Design review of the part built by this model. Coordinates are the model's own, in mm. Face numbers are marked on the shaded views. Give positions to 0.01 mm unless a question says otherwise; leave off trailing zeros. Order: outer loops, then holes, each group sorted by start corner. A loop starts at its lowest first (then second) coordinate and runs counter-clockwise, first axis right, second up. Notation, with made-up numbers: (61, 24.25) -> (100, 24.25) arc R22 cw to (100, 56.25) -> close; hole circle Ø11 at (65, 66.25). An arc over 180 degrees is marked (long way). Return JSON: item names as keys, results as strings.
```python
from build123d import *

# Parameters (mm, degrees)
SKETCH1_W           = 850
SKETCH1_H           = 450
BOSS_EXTRUDE1_DEPTH = 10
SKETCH2_W           = 50
SKETCH2_H           = 50
BOSS_EXTRUDE2_DEPTH = 675
BOSS_EXTRUDE3_REACH = 777
SKETCH3_W           = 13
SKETCH3_H           = 50
BOSS_EXTRUDE4_REACH = 377
SKETCH4_W           = 13
SKETCH4_H           = 50
SKETCH5_W           = 50
SKETCH5_H           = 25
BOSS_EXTRUDE5_DEPTH = 374
SKETCH6_W           = 50
SKETCH6_H           = 25
BOSS_EXTRUDE6_DEPTH = 374
LPATTERN2_COUNT     = 9
LPATTERN2_PITCH     = 80
LPATTERN3_COUNT     = 9
LPATTERN3_PITCH     = 80
CUT_EXTRUDE1_REACH  = 687
SKETCH7_R           = 150
FILLET2_R           = 5
FILLET3_R           = 5


with BuildPart() as part:
    # Sketch1 → Boss-Extrude1 (new body)
    with BuildSketch(Plane(origin=(0, 0, 0), x_dir=(1, 0, 0), z_dir=(0, 1, 0))):
        Rectangle(SKETCH1_W, SKETCH1_H)
    extrude(amount=BOSS_EXTRUDE1_DEPTH)

    # Sketch2 → Boss-Extrude2 (add)
    with BuildSketch(Plane.XZ):
        with Locations((-375, -175)):
            Rectangle(SKETCH2_W, SKETCH2_H)
        with Locations((-375, 175)):
            Rectangle(SKETCH2_W, SKETCH2_H)
        with Locations((375, 175)):
            Rectangle(SKETCH2_W, SKETCH2_H)
        with Locations((375, -175)):
            Rectangle(SKETCH2_W, SKETCH2_H)
    extrude(amount=BOSS_EXTRUDE2_DEPTH)

    # Sketch3 → Boss-Extrude3 (add, up to next)
    with BuildSketch(Plane(origin=(-350, 0, 0), x_dir=(0, 0, -1), z_dir=(1, 0, 0)), mode=Mode.PRIVATE) as boss_extrude3_sk1:
        with Locations((193.5, -600)):
            Rectangle(SKETCH3_W, SKETCH3_H)
    boss_extrude3_tool1 = extrude(boss_extrude3_sk1.sketch, amount=BOSS_EXTRUDE3_REACH, mode=Mode.PRIVATE) - part.part
    add(boss_extrude3_tool1.solids().sort_by_distance((-350, -600, -193.5))[0])
    # Sketch3 → Boss-Extrude3 (add, up to next)
    with BuildSketch(Plane(origin=(-350, 0, 0), x_dir=(0, 0, -1), z_dir=(1, 0, 0)), mode=Mode.PRIVATE) as boss_extrude3_sk2:
        with Locations((193.5, -325)):
            Rectangle(SKETCH3_W, SKETCH3_H)
    boss_extrude3_tool2 = extrude(boss_extrude3_sk2.sketch, amount=BOSS_EXTRUDE3_REACH, mode=Mode.PRIVATE) - part.part
    add(boss_extrude3_tool2.solids().sort_by_distance((-350, -325, -193.5))[0])
    # Sketch3 → Boss-Extrude3 (add, up to next)
    with BuildSketch(Plane(origin=(-350, 0, 0), x_dir=(0, 0, -1), z_dir=(1, 0, 0)), mode=Mode.PRIVATE) as boss_extrude3_sk3:
        with Locations((193.5, -25)):
            Rectangle(SKETCH3_W, SKETCH3_H)
    boss_extrude3_tool3 = extrude(boss_extrude3_sk3.sketch, amount=BOSS_EXTRUDE3_REACH, mode=Mode.PRIVATE) - part.part
    add(boss_extrude3_tool3.solids().sort_by_distance((-350, -25, -193.5))[0])

    # Mirror1: part across plane


with BuildPart() as part_1:
    add(part.part)
    add(part.part.mirror(Plane.XY))

    # Sketch4 → Boss-Extrude4 (add, up to next)
    with BuildSketch(Plane.XY.offset(-150), mode=Mode.PRIVATE) as boss_extrude4_sk1:
        with Locations((393.5, -600)):
            Rectangle(SKETCH4_W, SKETCH4_H)
    boss_extrude4_tool1 = extrude(boss_extrude4_sk1.sketch, amount=BOSS_EXTRUDE4_REACH, mode=Mode.PRIVATE) - part_1.part
    add(boss_extrude4_tool1.solids().sort_by_distance((393.5, -600, -150))[0])
    # Sketch4 → Boss-Extrude4 (add, up to next)
    with BuildSketch(Plane.XY.offset(-150), mode=Mode.PRIVATE) as boss_extrude4_sk2:
        with Locations((393.5, -325)):
            Rectangle(SKETCH4_W, SKETCH4_H)
    boss_extrude4_tool2 = extrude(boss_extrude4_sk2.sketch, amount=BOSS_EXTRUDE4_REACH, mode=Mode.PRIVATE) - part_1.part
    add(boss_extrude4_tool2.solids().sort_by_distance((393.5, -325, -150))[0])
    # Sketch4 → Boss-Extrude4 (add, up to next)
    with BuildSketch(Plane.XY.offset(-150), mode=Mode.PRIVATE) as boss_extrude4_sk3:
        with Locations((393.5, -25)):
            Rectangle(SKETCH4_W, SKETCH4_H)
    boss_extrude4_tool3 = extrude(boss_extrude4_sk3.sketch, amount=BOSS_EXTRUDE4_REACH, mode=Mode.PRIVATE) - part_1.part
    add(boss_extrude4_tool3.solids().sort_by_distance((393.5, -25, -150))[0])

    # Mirror2: part across plane


with BuildPart() as part_2:
    add(part_1.part)
    add(part_1.part.mirror(Plane(origin=(0, 0, 0), x_dir=(0, 0, 1), z_dir=(1, 0, 0))))

    # Sketch5 → Boss-Extrude5 (add)
    with BuildSketch(Plane.XY.offset(-187)):
        with Locations((-325, -337.5)):
            Rectangle(SKETCH5_W, SKETCH5_H)
    boss_extrude5 = extrude(amount=BOSS_EXTRUDE5_DEPTH)

    # Sketch6 → Boss-Extrude6 (add)
    with BuildSketch(Plane.XY.offset(-187)):
        with Locations((-325, -612.5)):
            Rectangle(SKETCH6_W, SKETCH6_H)
    boss_extrude6 = extrude(amount=BOSS_EXTRUDE6_DEPTH)

    # LPattern2: Boss-Extrude5 ×9
    with Locations(*[(i * LPATTERN2_PITCH, 0, 0) for i in range(1, LPATTERN2_COUNT)]):
        add(boss_extrude5)

    # LPattern3: Boss-Extrude6 ×9
    with Locations(*[(i * LPATTERN3_PITCH, 0, 0) for i in range(1, LPATTERN3_COUNT)]):
        add(boss_extrude6)

    # Sketch7 → Cut-Extrude1 (cut, up to next)
    with BuildSketch(Plane(origin=(0, 10, 0), x_dir=(1, 0, 0), z_dir=(0, 1, 0)), mode=Mode.PRIVATE) as cut_extrude1_sk1:
        with Locations((-225, 0)):
            Circle(SKETCH7_R)
    cut_extrude1_tool1 = extrude(cut_extrude1_sk1.sketch, amount=-CUT_EXTRUDE1_REACH, mode=Mode.PRIVATE) & part_2.part
    add(cut_extrude1_tool1.solids().sort_by_distance((-225, 10, 0))[0], mode=Mode.SUBTRACT)

    # Fillet2
    fillet2_edges = [part_2.edges().sort_by_distance(p)[0] for p in [
        (-400, -337.5, 200),
        (-350, -650, 200),
        (0, -625, 200),
        (350, -650, 200),
        (400, -337.5, 200),
        (0, -50, 200),
        (0, -300, 200),
        (0, -350, 200),
        (0, -575, 200),
        (-400, -175, -150),
        (-400, -300, 0),
        (-400, -175, 150),
        (-400, -50, 0),
        (-400, -462.5, -150),
        (-400, -575, 0),
        (-400, -462.5, 150),
        (-400, -350, 0),
        (-400, -650, -150),
        (-400, -337.5, -200),
        (400, -337.5, -200),
        (0, -625, -200),
        (0, -575, -200),
        (350, -462.5, -200),
        (0, -350, -200),
        (0, -300, -200),
        (400, -625, 0),
        (400, -462.5, 150),
        (400, -575, 0),
        (400, -350, 0),
        (400, -175, 150),
        (400, -300, 0),
        (400, -175, -150),
        (400, -50, 0),
        (-350, -650, 150),
        (350, -337.5, 150),
        (-350, -162.5, 150),
        (-350, -475, 150),
        (-350, -162.5, -150),
        (-350, -475, -150),
        (-350, -650, -150),
        (-387, -625, 0),
        (350, -337.5, -150),
        (0, -50, -187),
    ]]
    fillet(fillet2_edges, radius=FILLET2_R)

    # Fillet3
    fillet3_edges = [part_2.edges().sort_by_distance(p)[0] for p in [
        (-425, 10, 0),
        (0, 10, 225),
        (425, 10, 0),
        (0, 10, -225),
    ]]
    fillet(fillet3_edges, radius=FILLET3_R)


solid = part_2.part
```
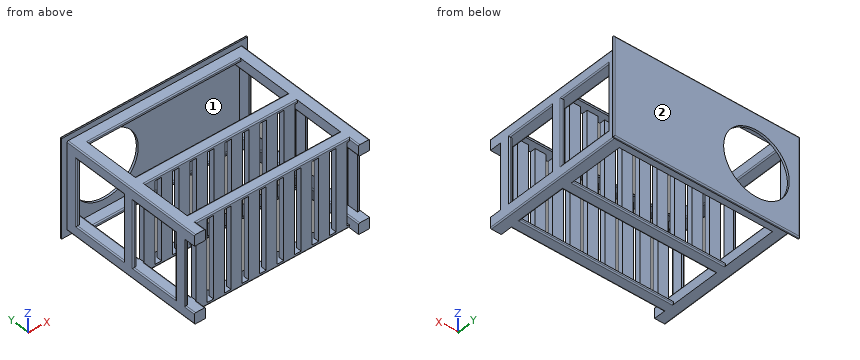
Item 1: Add section A-A (y = -279). Give the boundary of the cut face in (x, z).
Result set:
{"outline": "(-400, -195) arc R5 ccw to (-395, -200) -> (-350, -200) -> (-350, -155) arc R5 ccw to (-355, -150) -> (-395, -150) arc R5 ccw to (-400, -155) -> close; (-400, 155) arc R5 ccw to (-395, 150) -> (-355, 150) arc R5 ccw to (-350, 155) -> (-350, 200) -> (-395, 200) arc R5 ccw to (-400, 195) -> close; (350, -200) -> (395, -200) arc R5 ccw to (400, -195) -> (400, -155) arc R5 ccw to (395, -150) -> (355, -150) arc R5 ccw to (350, -155) -> close; (350, 155) arc R5 ccw to (355, 150) -> (395, 150) arc R5 ccw to (400, 155) -> (400, 195) arc R5 ccw to (395, 200) -> (350, 200) -> close"}
Item 2: Mouldability with a two-part tool opening along Y and no side actions: class the marked faces 1 and 2 as released by +Y, released by -Y, zero draft, split by the parting line, or undercut.
Result set:
{"face 1": "undercut", "face 2": "released by +Y"}
Item 3: Add section B-B (z = 0). Give the number of separate pieces and of enclosed holes in the cut face, plus the area to 3 significant figures.
Result set:
{"separate pieces": "24", "enclosed holes": "0", "area": "31,800 mm^2"}
Item 4: For pin 1 (12.5 mm diameter, centred on y = -610, z = -56.5, fed in from -X); pin 2 (20 mm diameter, centred on y = -614, z = 67.5, fed in from +X); pin 3 (2.5 mm diameter, centred on x = -392, z = -20, fed in from -Y), all flat-tipped, find the tip position at first contact; note any pin that passes through.
Result set:
{"pin 1": "stops at x = -400", "pin 2": "stops at x = 400", "pin 3": "stops at y = -625"}
Item 5: Wall thickness on L1, parallel to Y at x = 251.5, z = -150.5; L2, parallel to X at y = 6, z = 0; L3, parallel to Z at x = -225, y = 4.75: over which ranges is each line inside the solid? List them lowest first. Write a range as [from, to].
Result set:
{"L1": "y = [-625, -600], [-350, -325], [0, 10]", "L2": "x = [-424.9, -375], [-75, 424.9]", "L3": "z = [-225, -150], [150, 225]"}
